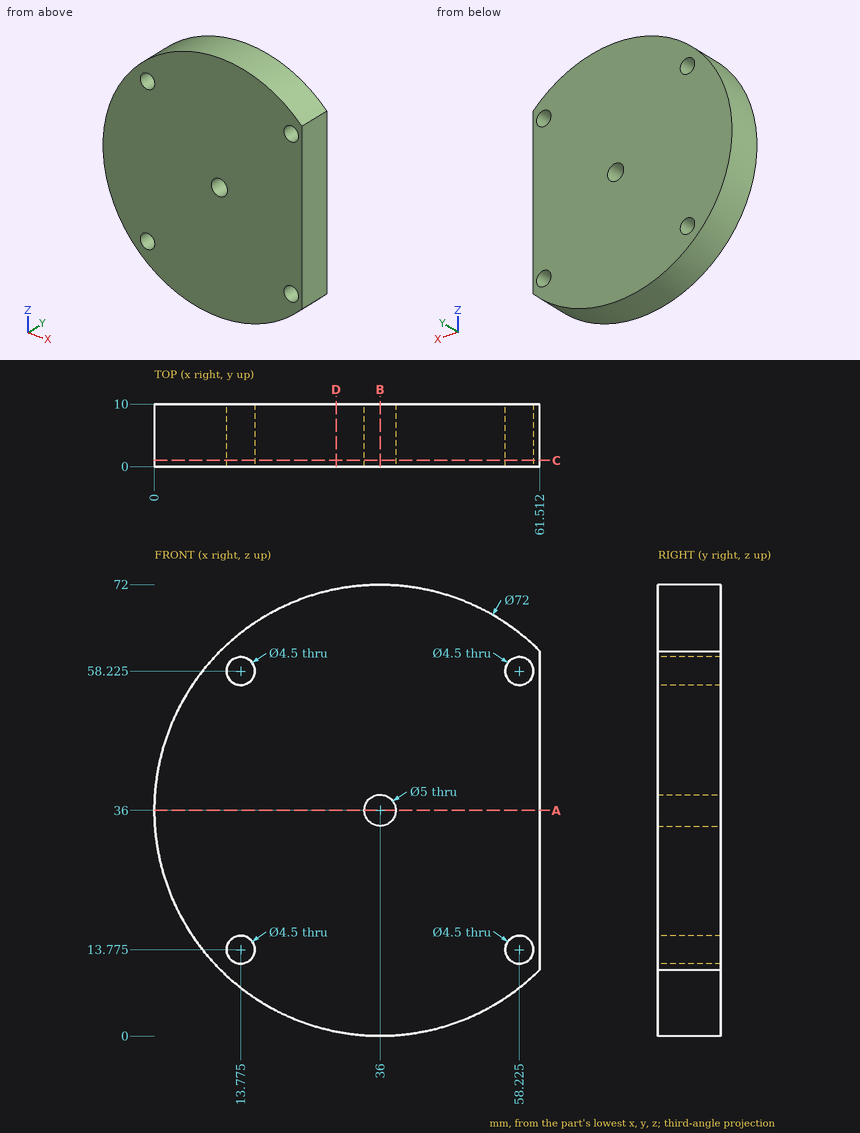
Could you check a few things on this drawing? It's one solid part, dimensions in mm from its lowest x, y, z. Round coordinates to 2 decimals unless told otherwise and drop trailing zeros. Order: outer loops, then holes, each group sorted by start corner. A loop starts at its lowest first (then second) coordinate and runs counter-clockwise, first axis right, second up. Notation, with made-up numbers: M 0,47.5 L 20,47.5 A25 ccw 20,80.5 Z; hole C 67.5,5 d11. An arc over 180 degrees is marked long. One line per question, with ' | ' between items. Start each with the question number.
(1) Suppose I cut it at B-B on x = 36. List the corners of the cut face in (y, z) for me, then the cut area to 3 significant figures.
(2) Suppose I cut it at D-D on x = 29. List the corners of the cut face in (y, z) for me.
(3) Suppose I cut it at A-A on z = 36. List the corners of the cut face in (x, y) for me.
(4) Please list where these lines run through material, in increasing order: line 1 along X through (y, z) = (2.75, 58); line 2 along Z through (x, y) = (58.5, 2); line 3 along Z through (x, y) = (15, 3.25).
(5) For P1, Ø3, axis at y = 6, z = 58.5, coming from the -X side; P2, Ø2.5, axis at x = 13.775, z = 13.775, coming from the +Y side; P3, Ø6, axis at x = 55, y = 4.5, coming from the -Z side; P4, Ø4, axis at y = 4.5, z = 20.5, coming from the -X side, each with a flat end and sliding along its axis, tell me the tip position at first contact or that it passes through.
(6) Suppose I cut it at C-C on y = 1. List the corners of the cut face in (x, z) for me (3 decimals).
Geometry results:
1) outline: M 0,0 L 10,0 L 10,33.5 L 0,33.5 Z; M 0,38.5 L 10,38.5 L 10,72 L 0,72 Z | area: 670 mm²
2) outline: M 0,0.69 L 10,0.69 L 10,71.31 L 0,71.31 Z
3) outline: M 0,0 L 33.5,0 L 33.5,10 L 0,10 Z; M 38.5,0 L 61.51,0 L 61.51,10 L 38.5,10 Z
4) line 1: 7.5 to 11.54, 16.01 to 55.99, 60.46 to 61.51 | line 2: 7.9 to 11.54, 16.01 to 55.99, 60.46 to 64.1 | line 3: 6.76 to 11.89, 15.66 to 56.34, 60.11 to 65.24
5) P1: x = 6.76 | P2: through | P3: z = 3.75 | P4: x = 2.63
6) outline: M 61.512,10.6 L 61.512,61.4 A36 ccw long Z; hole C 13.775,13.775 d4.5; hole C 13.775,58.225 d4.5; hole C 36,36 d5; hole C 58.225,13.775 d4.5; hole C 58.225,58.225 d4.5
